Source: CAD feature listing. Evaluate the final solid. Frame: model axes, mm. A direction names the side the tool comes from. Give positions to 0.01 mm unless a question says otherwise; leave off trailing zeros. Order: outer loops, then holes, each group sorted by start corner. A loop starts at its lowest first (then second) coordinate and runs counter-clockwise, first axis right, second up. Notation, with made-up numbers: (74, -21.75) - (126, -21.75) arc R11 cw to (126, -12.75) - close; hole circle Ø11 at (71, 40). An arc over 180 degrees is marked (long way). Write each question's results on one line, items separated by ' | '. Start each with the question number.
Item 1: Line query: line 1 along Z through (x, y) = (25, 26.5); line 2 along Z through (x, y) = (32.75, 29); line 3 along Y through (x, z) = (29, 52.25). Output: solid intervals per line, ascending.
Item 2: Section B-B on y = 56. Output: boundary loops of the cut face in (x, z) (3 decimals).
Item 3: Set-up query: faces 4 (the cylindrical face through (25.99, 16.96, 51.84)), 5 (the flat face through (28, 48, 38)), 6 (the flat face through (28, 20, 39)), 7 (the cylindrical face through (25.99, 6.96, 24.88)), 8 (the flat face through (25, 23, 35.86)). Return all of +Z, -Z, +X, -X, +Y, -Y with unobstructed straight access to the full face (end or side cutting, diameter ignored); none if empty.
Item 4: Section C-C on z = 39.75. Output: boundary loops of the cut face in (x, y), and give its area (3 significant figures).
Item 5: Mould query, pull axis Z, two halves, no side actions, for faces 1 (the cylindrical face through (25.99, 6.96, 51.84)), 2 (the flat face through (28, 6, 23.36)), 3 (the flat face through (28, 18, 36.11)). Classes: released by +Z, released by -Z, zero draft, split by the parting line, or undercut.
Item 6: Contact query for flat-ended pins moving along their axis: pin 1 Ø1.1 at (x, z) = (24, 41.5) entering from -Y; pin 2 Ø0.6 at (x, y) = (24.5, 24.5) entering from -Z; pin 3 Ø2 at (x, y) = (30.5, 29) entering from +Z. Output: stop coordinate, or through.
Item 7: Section A-A on y = 6. Output: boundary loops of the cut face in (x, z), and give its area (3 significant figures).
Item 8: Section D-D on y = 23. Output: boundary loops of the cut face in (x, z).
```python
from build123d import *

# Parameters (mm, degrees)
SKETCH1_W               = 9.25
SKETCH1_H               = 20
BOSS_EXTRUDE1_DEPTH     = 70
SKETCH2_R               = 2.625
CUT_EXTRUDE1_DEPTH      = 22
SKETCH4_R               = 5.5
CUT_EXTRUDE3_DEPTH      = 20
SKETCH5_W               = 2.148979486
SKETCH5_H               = 5
CUT_EXTRUDE4_DEPTH      = 7
CUT_EXTRUDE5_DEPTH      = 86.328689654
CUT_EXTRUDE5_DEPTH_BACK = 4
SKETCH6_W               = 4.5
SKETCH6_H               = 4
SKETCH7_R               = 2.5
BOSS_EXTRUDE2_DEPTH     = 5
FILLET1_R               = 2


with BuildPart() as part:
    # Sketch1 → Boss-Extrude1 (new body)
    with BuildSketch(Plane(origin=(0, 0, 0), x_dir=(1, 0, 0), z_dir=(0, 1, 0))):
        with Locations((28.297124636, -38.360472269)):
            Rectangle(SKETCH1_W, SKETCH1_H)
    extrude(amount=BOSS_EXTRUDE1_DEPTH)

    # Sketch2 → Cut-Extrude1 (cut)
    with BuildSketch(Plane(origin=(0, 70, 0), x_dir=(1, 0, 0), z_dir=(0, 1, 0))):
        with Locations(Location((28.297124636, -38.360472269, 0), (0, 0, 270))):
            Circle(SKETCH2_R)
    extrude(amount=-CUT_EXTRUDE1_DEPTH, mode=Mode.SUBTRACT)

    # Sketch4 → Cut-Extrude3 (cut)
    with BuildSketch(Plane(origin=(0, 0, 0), x_dir=(-1, 0, 0), z_dir=(0, -1, 0))):
        with Locations((-20.922124636, -38.360472269)):
            Circle(SKETCH4_R)
    extrude(amount=-CUT_EXTRUDE3_DEPTH, mode=Mode.SUBTRACT)

    # Sketch5 → Cut-Extrude4 (cut)
    with BuildSketch(Plane(origin=(0, 20, 0), x_dir=(-1, 0, 0), z_dir=(0, -1, 0))):
        with Locations((-24.746614379, -38.360472269)):
            Rectangle(SKETCH5_W, SKETCH5_H)
    extrude(amount=-CUT_EXTRUDE4_DEPTH, mode=Mode.SUBTRACT)

    # Sketch6 → Cut-Extrude5 (cut, two sides: drawn at the far end of the back side and taken through both)
    with BuildSketch(Plane.ZY.offset(-26.422124636).offset(-CUT_EXTRUDE5_DEPTH_BACK)):
        with Locations((38.360472269, 18)):
            Rectangle(SKETCH6_W, SKETCH6_H)
    extrude(amount=CUT_EXTRUDE5_DEPTH + CUT_EXTRUDE5_DEPTH_BACK, mode=Mode.SUBTRACT)

    # Sketch7 → Boss-Extrude2 (add)
    with BuildSketch(Plane.XY.offset(48.360472269)):
        with Locations(Location((28.297124636, 6, 0), (0, 0, 180))):
            Circle(SKETCH7_R)
        with Locations(Location((28.297124636, 16, 0), (0, 0, 180))):
            Circle(SKETCH7_R)
    boss_extrude2 = extrude(amount=BOSS_EXTRUDE2_DEPTH)

    # Mirror1: Boss-Extrude2 across plane
    add(boss_extrude2.mirror(Plane(origin=(0, 0, 38.360472269), x_dir=(1, 0, 0), z_dir=(0, 0, -1))))

    # Fillet1
    fillet1_edges = [part.edges().sort_by_distance(p)[0] for p in [
        (30.797124636, 6, 48.360472269),
        (30.797124636, 16, 48.360472269),
        (30.797124636, 6, 28.360472269),
        (30.797124636, 16, 28.360472269),
    ]]
    fillet(fillet1_edges, radius=FILLET1_R)


solid = part.part
```
Evaluation:
1) line 1: z = 28.36 to 35.86, 40.86 to 48.36 | line 2: z = 28.36 to 48.36 | line 3: y = 3.6 to 8.4, 13.6 to 18.4
2) outline: (23.672, 28.36) - (32.922, 28.36) - (32.922, 48.36) - (23.672, 48.36) - close; hole circle Ø5.25 at (28.297, 38.36)
3) face 4: +Z | face 5: +Y | face 6: -X | face 7: -Z | face 8: -X, -Y
4) outline: (23.67, 27) - (25.82, 27) - (25.82, 20) - (30.42, 20) - (30.42, 16) - (26.24, 16) - (26.24, 0) - (32.92, 0) - (32.92, 70) - (30.52, 70) - (30.52, 48) - (26.07, 48) - (26.07, 70) - (23.67, 70) - close | area: 466 mm^2
5) face 1: zero draft | face 2: released by -Z | face 3: undercut
6) pin 1: stops at y = 20 | pin 2: stops at z = 28.36 | pin 3: stops at z = 48.36
7) outline: (23.67, 28.36) - (23.8, 28.36) arc R2 cw to (25.8, 26.36) - (25.8, 23.36) - (30.8, 23.36) - (30.8, 26.36) arc R2 cw to (32.8, 28.36) - (32.92, 28.36) - (32.92, 48.36) - (32.8, 48.36) arc R2 cw to (30.8, 50.36) - (30.8, 53.36) - (25.8, 53.36) - (25.8, 50.36) arc R2 cw to (23.8, 48.36) - (23.67, 48.36) - (23.67, 43.12) arc R5.5 cw to (23.67, 33.6) - close | area: 220 mm^2
8) outline: (23.67, 28.36) - (32.92, 28.36) - (32.92, 48.36) - (23.67, 48.36) - (23.67, 40.86) - (25.82, 40.86) - (25.82, 35.86) - (23.67, 35.86) - close
